Input: part model. Units: mm. Frame: model coordinates. Round coordinates to 2 decimals unless told otherwise and drop trailing zeros. Loops run counter-clockwise (first coordinate to the right, second up) from the corner with the lowest first, then second, coordinate; pieces in that order, holes last.
1) Ray query, line 1 along X through (y, z) = (1.6, -16) (3 decimals); line 2 along Z through (x, y) = (-37.5, 1.05) (3 decimals); line 3 along X through (y, z) = (2.65, 0). Return the intervals inside material, ascending.
2) Section A-A, the plane y = 2.4. Return loops of the section in (x, z) (3 decimals), and give its area (3 significant figures).
3) Section C-C, the plane z = 16. Return loops of the section in (x, y) (3 decimals).
4) First-contact query: pin 1 (0.8 mm diameter, centred on x = -40, y = 3, fed in from -Z); pin 2 (1.3 mm diameter, centred on y = 3, z = 18, fed in from +X). Flat tips, straight axial feed; report the tip coordinate or a pass-through.
5) Section B-B, the plane x = -37.5. Return loops of the section in (y, z) (3 decimals).
6) Section D-D, the plane x = 41. Return loops of the section in (y, z) (3 decimals).
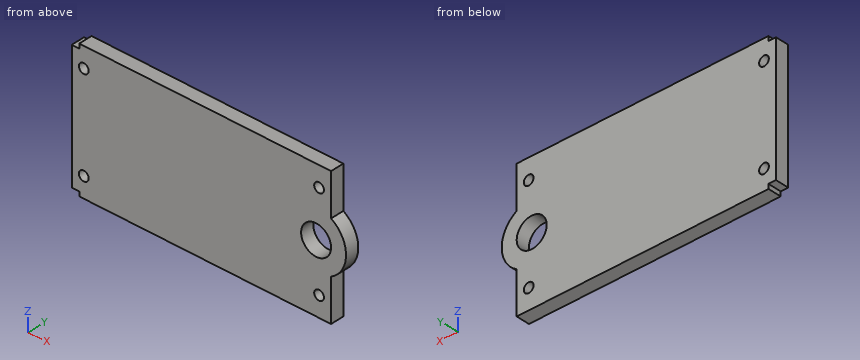
from build123d import *

# Parameters (mm, degrees)
SKETCH2_W           = 86.5
SKETCH2_H           = 45.5
BOSS_EXTRUDE1_DEPTH = 4.5
SKETCH3_R           = 1.625
CUT_EXTRUDE1_DEPTH  = 5.5
SKETCH5_R           = 10
BOSS_EXTRUDE2_DEPTH = 4.5
SKETCH6_R           = 5
CUT_EXTRUDE3_DEPTH  = 5.5
SKETCH7_W           = 2.5
SKETCH7_H           = 1.5
CUT_EXTRUDE4_DEPTH  = 5.5


with BuildPart() as part:
    # Sketch2 → Boss-Extrude1 (new body)
    with BuildSketch(Plane(origin=(0, 0, 0), x_dir=(1, 0, 0), z_dir=(0, 1, 0))):
        with Locations((1.75, 0)):
            Rectangle(SKETCH2_W, SKETCH2_H)
    extrude(amount=BOSS_EXTRUDE1_DEPTH)

    # Sketch3 → Cut-Extrude1 (cut, through all)
    with BuildSketch(Plane(origin=(0, 4.5, 0), x_dir=(1, 0, 0), z_dir=(0, 1, 0))):
        with Locations((-37.5, -16)):
            Circle(SKETCH3_R)
        with Locations((-37.5, 16)):
            Circle(SKETCH3_R)
        with Locations((41, 16)):
            Circle(SKETCH3_R)
        with Locations((41, -16)):
            Circle(SKETCH3_R)
    extrude(amount=-CUT_EXTRUDE1_DEPTH, mode=Mode.SUBTRACT)

    # Sketch5 → Boss-Extrude2 (add)
    with BuildSketch(Plane(origin=(0, 4.5, 0), x_dir=(1, 0, 0), z_dir=(0, 1, 0))):
        with Locations((40, 0)):
            Circle(SKETCH5_R)
    extrude(amount=-BOSS_EXTRUDE2_DEPTH)

    # Sketch6 → Cut-Extrude3 (cut, through all)
    with BuildSketch(Plane(origin=(0, 4.5, 0), x_dir=(1, 0, 0), z_dir=(0, 1, 0))):
        with Locations((40, 0)):
            Circle(SKETCH6_R)
    extrude(amount=-CUT_EXTRUDE3_DEPTH, mode=Mode.SUBTRACT)

    # Sketch7 → Cut-Extrude4 (cut, through all)
    with BuildSketch(Plane(origin=(0, 4.5, 0), x_dir=(1, 0, 0), z_dir=(0, 1, 0))):
        with Locations((-40.25, 22)):
            Rectangle(SKETCH7_W, SKETCH7_H)
        with Locations((-40.25, -22)):
            Rectangle(SKETCH7_W, SKETCH7_H)
    extrude(amount=-CUT_EXTRUDE4_DEPTH, mode=Mode.SUBTRACT)


solid = part.part
Final values:
1. line 1: x = -41.5 to -39.125, -35.875 to 39.375, 42.625 to 45
1. line 2: z = -22.75 to -17.625, -14.375 to 14.375, 17.625 to 22.75
1. line 3: x = -41.5 to 35, 45 to 50
2. outline: (-41.5, -21.25) - (-39, -21.25) - (-39, -22.75) - (45, -22.75) - (45, -8.66) arc R10 ccw to (45, 8.66) - (45, 22.75) - (-39, 22.75) - (-39, 21.25) - (-41.5, 21.25) - close; hole circle Ø3.25 at (-37.5, -16); hole circle Ø3.25 at (-37.5, 16); hole circle Ø10 at (40, 0); hole circle Ø3.25 at (41, -16); hole circle Ø3.25 at (41, 16)
2. area: 3,880 mm2
3. outline: (-41.5, 0) - (-39.125, 0) - (-39.125, 4.5) - (-41.5, 4.5) - close; (-35.875, 0) - (39.375, 0) - (39.375, 4.5) - (-35.875, 4.5) - close; (42.625, 0) - (45, 0) - (45, 4.5) - (42.625, 4.5) - close
4. pin 1: stops at z = -21.25
4. pin 2: stops at x = 45
5. outline: (0, -22.75) - (4.5, -22.75) - (4.5, -17.625) - (0, -17.625) - close; (0, -14.375) - (4.5, -14.375) - (4.5, 14.375) - (0, 14.375) - close; (0, 17.625) - (4.5, 17.625) - (4.5, 22.75) - (0, 22.75) - close
6. outline: (0, -22.75) - (4.5, -22.75) - (4.5, -17.625) - (0, -17.625) - close; (0, -14.375) - (4.5, -14.375) - (4.5, -4.899) - (0, -4.899) - close; (0, 4.899) - (4.5, 4.899) - (4.5, 14.375) - (0, 14.375) - close; (0, 17.625) - (4.5, 17.625) - (4.5, 22.75) - (0, 22.75) - close
